Check sheet for the modelled part. Datum: model origin and axes. Units: mm. A direction names the side the tool comes from. Give positions to 0.01 mm unless a question says otherwise; leave off trailing zeros. Order: outer loops, then holes, each group sorted by start corner. A loop starts at its lowest first (then second) coordinate and runs counter-clockwise, first axis right, second up.
Item 1: Gauge pin test, flat ends, axial feed: P1, Ø5, axis at x = 7, z = 24, coming from the -Y side; P2, Ø6, axis at x = 4.5, z = 21, coming from the +Y side; P3, Ø10, axis at y = 5.5, z = 17, coming from the -X side. Record the tip position at first contact, or that the pin passes through.
Item 2: Release check for a two-part mould opening along Y. For faces 3 (the flat face through (5, -5, 30)), 4 (the cylindrical face through (10, 3.2, 14.9)), 5 (the cylindrical face through (-6, 0, 15)) record: released by +Y, released by -Y, zero draft, split by the parting line, or undercut.
Item 3: Sectioned sample at D-D on x = -9. Record the boundary of the cut face in (y, z), and give its area (3 significant figures).
Item 4: Access from +Z, -Z, +X, -X, +Y, -Y to the whole of each face (thin tool, end or side, straight path). Record for faces 1 (the flat face through (9, -5, 3.5)), 2 (the cylindrical face through (10, 3.2, 1.7)).
Item 5: Material ranges on line 1 along Z through (x, y) = (7.25, 7); line 2 along Y through (x, z) = (-5, 5.5); line 3 along Y through (x, z) = (4.75, 13), recorded low to high.
Item 6: Sectioned sample at C-C on z = 12.5. Record the boundary of the cut face in (x, y).
Item 7: Sectioned sample at A-A on x = 0. Record the boundary of the cut face in (y, z), and give its area (3 significant figures).
from build123d import *

# Parameters (mm, degrees)
ESBO_O1_R                  = 10.5
RESSALTO_EXTRUS_O1_DEPTH   = 30
ESBO_O2_R                  = 6
CORTE_EXTRUS_O1_DEPTH      = 1
CORTE_EXTRUS_O1_DEPTH_BACK = 31
ESBO_O4_W                  = 1.3
ESBO_O4_H                  = 0.5


with BuildPart() as part:
    # Esboço1 → Ressalto-extrusão1 (new body)
    with BuildSketch(Plane.XY):
        Circle(ESBO_O1_R)
    extrude(amount=RESSALTO_EXTRUS_O1_DEPTH)

    # Esboço2 → Corte-extrusão1 (cut, two sides)
    with BuildSketch(Plane.XY.offset(30)) as corte_extrus_o1_sk:
        Circle(ESBO_O2_R)
    extrude(amount=CORTE_EXTRUS_O1_DEPTH, mode=Mode.SUBTRACT)
    extrude(corte_extrus_o1_sk.sketch, amount=-CORTE_EXTRUS_O1_DEPTH_BACK, mode=Mode.SUBTRACT)

    # Esboço4 → Corte-Revolução1 (revolve, cut)
    with BuildSketch(Plane(origin=(0, 0, 0), x_dir=(0, 0, -1), z_dir=(1, 0, 0))):
        with Locations((-25.85, 10.25)):
            Rectangle(ESBO_O4_W, ESBO_O4_H)
        with Locations((-4.15, 10.25)):
            Rectangle(ESBO_O4_W, ESBO_O4_H)
    revolve(axis=Axis((0, 0, -1.457000242), (0, 0, 1)), mode=Mode.SUBTRACT)


solid = part.part
Report:
1. P1: stops at y = -9.49
1. P2: stops at y = 10.39
1. P3: stops at x = -10.49
2. face 3: zero draft
2. face 4: split by the parting line
2. face 5: undercut
3. outline: (-5.41, 0) - (5.41, 0) - (5.41, 3.5) - (4.36, 3.5) - (4.36, 4.8) - (5.41, 4.8) - (5.41, 25.2) - (4.36, 25.2) - (4.36, 26.5) - (5.41, 26.5) - (5.41, 30) - (-5.41, 30) - (-5.41, 26.5) - (-4.36, 26.5) - (-4.36, 25.2) - (-5.41, 25.2) - (-5.41, 4.8) - (-4.36, 4.8) - (-4.36, 3.5) - (-5.41, 3.5) - close
3. area: 319 mm2
4. face 1: none
4. face 2: +Z, -Z
5. line 1: z = 0 to 3.5, 4.8 to 25.2, 26.5 to 30
5. line 2: y = -9.23 to -3.32, 3.32 to 9.23
5. line 3: y = -9.36 to -3.67, 3.67 to 9.36
6. outline: circle Ø21 at (0, 0); hole circle Ø12 at (0, 0)
7. outline: (-10.5, 0) - (-6, 0) - (-6, 30) - (-10.5, 30) - (-10.5, 26.5) - (-10, 26.5) - (-10, 25.2) - (-10.5, 25.2) - (-10.5, 4.8) - (-10, 4.8) - (-10, 3.5) - (-10.5, 3.5) - close; (6, 0) - (10.5, 0) - (10.5, 3.5) - (10, 3.5) - (10, 4.8) - (10.5, 4.8) - (10.5, 25.2) - (10, 25.2) - (10, 26.5) - (10.5, 26.5) - (10.5, 30) - (6, 30) - close
7. area: 267 mm2
